```python
from build123d import *

# Parameters (mm, degrees)
F0_R     = 38.1
F1_DEPTH = 25.4
F2_W     = 44.03428
F2_H     = 85.478309
F3_DEPTH = 25.4
F4_R     = 5.08


with BuildPart() as f1:
    # F0 (on Top) → F1 (new body)
    with BuildSketch(Plane.XY):
        Circle(F0_R)
    extrude(amount=F1_DEPTH)

    # F2 (on face) → F3 (cut)
    with BuildSketch(Plane.XY.offset(25.4)):
        with Locations((22.01714, -1.870739)):
            Rectangle(F2_W, F2_H)
    extrude(amount=-F3_DEPTH, mode=Mode.SUBTRACT)

    # F4
    f4_edges = [f1.edges().sort_by_distance(p)[0] for p in [
        (0, 0, 25.4),
        (0, -38.1, 12.7),
        (0, 38.1, 12.7),
        (-38.1, 0, 25.4),
        (-38.1, 0, 0),
        (0, 0, 0),
    ]]
    fillet(f4_edges, radius=F4_R)


solid = f1.part
```
Here's how the part is built. I have some questions about the finished solid (model axes, mm). Give positions to 0.01 mm unless a question says otherwise; leave off trailing zeros. Order: outer loops, then holes, each group sorted by start corner. A loop starts at its lowest first (then second) coordinate and runs counter-clockwise, first axis right, second up. Notation, with made-up numbers: M 70.25,82.5 L 112.25,82.5 A13 ccw 112.25,98.5 Z; hole C -2.75,-8 d4. An arc over 180 degrees is marked long. Use a Markdown table: item, result. Add a question column.
1. Suppose I cut it at B-B (z = 14.5). List the corners of the cut face in (x, y) for me.
2. For pin 1 Ø2 at (x, z) = (-21, 13) entering from +Y; pin 2 Ø3 at (y, z) = (12, 2.5) entering from +X; pin 3 Ø2 at (y, z) = (-28, 8.5) entering from -X, each with a flat end and sliding along its axis, tell me the tip position at first contact or that it passes through.
3. Suppose I cut it at A-A (x = -3.5). List the corners of the cut face in (y, z) for me, and give its area (3 significant figures).
4. I need wall thicknesses on probe 1 along X at (y, z) = (1, 7.25); probe 2 along Z at (x, y) = (-2, -16); probe 3 along X at (y, z) = (-6, 23.5). Which ranges of each line are inside material? Lowest first, please. Write a range as from..to.
5. Suppose I cut it at C-C (z = 22.25). List the corners of the cut face in (x, y) for me.
Results list:
| question | item | result |
|---|---|---|
| 1 | outline | M -5.86,-37.65 A5.08 ccw 0,-32.63 L 0,32.63 A5.08 ccw -5.86,37.65 A38.1 ccw Z |
| 2 | pin 1 | stops at y = 32.43 |
| 2 | pin 2 | stops at x = -0.12 |
| 2 | pin 3 | stops at x = -26.88 |
| 3 | outline | M -37.45,5.08 A4.83 ccw -32.63,0.25 L 32.63,0.25 A4.83 ccw 37.45,5.08 L 37.45,20.32 A4.83 ccw 32.63,25.15 L -32.63,25.15 A4.83 ccw -37.45,20.32 Z |
| 3 | area | 1,840 mm² |
| 4 | probe 1 | x = -38.09..0 |
| 4 | probe 2 | z = 1.04..24.36 |
| 4 | probe 3 | x = -36.49..-1.12 |
| 5 | outline | M -5.8,-37.27 A4.7 ccw -0.38,-32.63 L -0.38,32.63 A4.7 ccw -5.8,37.27 A37.72 ccw Z |
